Could you check a few things on this model? Use its own coordinates, in mm. Face numbers are marked on the shaded views. A direction names the side the tool comes from. Round coordinates to 2 decimals unless told otherwise and drop trailing zeros. Loops run counter-clockwise (first coordinate to the right, second up) from the corner with the lowest first, then second, coordinate; pieces in that order, holes last.
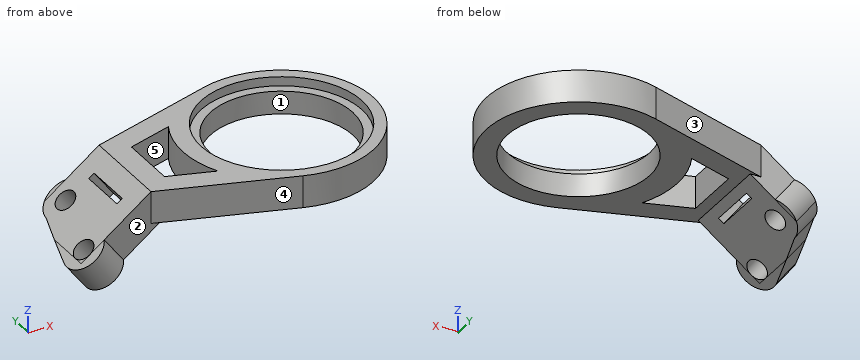
from build123d import *

# Parameters (mm, degrees)
SKETCH_1_R           = 7.75
EXTRUDE_1_DEPTH      = 3.5
SKETCH_2_R           = 8.75
CUT_EXTRUDE_1_DEPTH  = 1
EXTRUDE_2_DEPTH      = 5
SKETCH_8_W           = 0.720416832
SKETCH_8_H           = 5.4
CUT_EXTRUDE_6_DEPTH  = 26.612556655
EXTRUDE_6_DEPTH      = 3.5
SKETCH_4_9_R         = 1.15
CUT_EXTRUDE_9_DEPTH  = 27.034467236
CUT_EXTRUDE_10_DEPTH = 3.5


with BuildPart() as part:
    # 草图1 → 凸台-拉伸1 (new body)
    with BuildSketch(Plane.XY):
        with BuildLine():
            Line((-3.074847287, 9.515530157), (-17.048765133, 5))
            Line((-17.048765133, 5), (-17.048765133, -5))
            Line((-17.048765133, -5), (-3.074847287, -9.515530157))
            ThreePointArc((-3.074847287, -9.515530157), (10, 0), (-3.074847287, 9.515530157))
        make_face()
        Circle(SKETCH_1_R, mode=Mode.SUBTRACT)
        with BuildLine():
            Line((-14.548765133, 3.180565718), (-14.548765133, -3.180565718))
            Line((-14.548765133, -3.180565718), (-9.63448381, -4.768566002))
            ThreePointArc((-9.63448381, -4.768566002), (-10.75, 0), (-9.63448381, 4.768566002))
            Line((-9.63448381, 4.768566002), (-14.548765133, 3.180565718))
        make_face(mode=Mode.SUBTRACT)
    extrude(amount=EXTRUDE_1_DEPTH)

    # 草图2 → 切除-拉伸1 (cut)
    with BuildSketch(Plane.XY.offset(3.5)):
        Circle(SKETCH_2_R)
    extrude(amount=-CUT_EXTRUDE_1_DEPTH, mode=Mode.SUBTRACT)

    # 草图3 → 凸台-拉伸2 (add, symmetric)
    with BuildSketch(Plane(origin=(0, 0, 0), x_dir=(1, 0, 0), z_dir=(0, 1, 0))):
        Polygon((-17.048765133, -3.5), (-24.66318775, 2.214797011), (-22.562251427, 5.014094523), (-15.881448124, 0), align=None)
    extrude(amount=EXTRUDE_2_DEPTH, both=True)

    # 草图8 → 切除-拉伸6 (cut, through all)
    with BuildSketch(Plane(origin=(-7.82335713, 0, 10.423878111), x_dir=(0.7997992893547787, 0, 0.6002675209834286), z_dir=(-0.6002675209834286, 0, 0.7997992893547787))):
        with Locations((-14.194862331, 0)):
            Rectangle(SKETCH_8_W, SKETCH_8_H)
    extrude(amount=-CUT_EXTRUDE_6_DEPTH, mode=Mode.SUBTRACT)

    # 草图4 → 凸台-拉伸6 (add)
    with BuildSketch(Plane(origin=(-7.82335713, 0, 10.423878111), x_dir=(0.7997992893547787, 0, 0.6002675209834286), z_dir=(-0.6002675209834286, 0, 0.7997992893547787))):
        with BuildLine():
            Line((-19.939913719, 3.705712142), (-22.099126281, -3.159985282))
            ThreePointArc((-22.099126281, -3.159985282), (-20.830616239, -5.955555875), (-17.913212318, -5))
            Line((-17.913212318, -5), (-17.348837919, 1.241173708))
            Line((-17.348837919, 1.241173708), (-16.116035743, 2.269506831))
            Line((-16.116035743, 2.269506831), (-16.116035743, 5))
            ThreePointArc((-16.116035743, 5), (-18.356590206, 5.323726244), (-19.939913719, 3.705712142))
        make_face()
    extrude(amount=-EXTRUDE_6_DEPTH)

    # 草图4<9> → 切除-拉伸9 (cut, through all)
    with BuildSketch(Plane(origin=(-7.82335713, 0, 10.423878111), x_dir=(0.7997992893547787, 0, 0.6002675209834286), z_dir=(-0.6002675209834286, 0, 0.7997992893547787))):
        with Locations((-17.555070747, 2.955696144)):
            Circle(SKETCH_4_9_R)
        with Locations((-19.905070747, -3.85)):
            Circle(SKETCH_4_9_R)
    extrude(amount=-CUT_EXTRUDE_9_DEPTH, mode=Mode.SUBTRACT)

    # 草图9 → 切除-拉伸10 (cut)
    with BuildSketch(Plane(origin=(-7.82335713, 0, 10.423878111), x_dir=(0.7997992893547787, 0, 0.6002675209834286), z_dir=(-0.6002675209834286, 0, 0.7997992893547787))):
        with BuildLine():
            Line((-21.055070747, 0.15982191), (-20.046766168, 3.15929852))
            ThreePointArc((-20.046766168, 3.15929852), (-19.725256431, 4.196781997), (-18.994105751, 5))
            Line((-18.994105751, 5), (-18.994105751, 5.471830363))
            Line((-18.994105751, 5.471830363), (-21.906262893, 5.471830363))
            Line((-21.906262893, 5.471830363), (-21.906262893, 0.15982191))
            Line((-21.906262893, 0.15982191), (-21.055070747, 0.15982191))
        make_face()
    extrude(amount=-CUT_EXTRUDE_10_DEPTH, mode=Mode.SUBTRACT)


solid = part.part
Item 1: If I drill on line 1 along X through (y, z) = (0, 2.05); line 2 along Y through (x, z) = (0, 1); line 3 along X through (y, z) = (0.75, 1.5), over which ranges is the centre line in solid material (lowest first)?
Results list:
line 1: x = -18.84 to -14.55, -10.75 to -7.75, 7.75 to 10
line 2: y = -10 to -7.75, 7.75 to 10
line 3: x = -19.71 to -19.32, -18.42 to -14.55, -10.72 to -7.71, 7.71 to 9.97
Item 2: Will these pins go through, and if not, where does the flat tip stop? pin 1 (6 mm diameter, centred on x = -8.5, y = 3.5, fed in from -Z); pin 2 (3 mm diameter, centred on x = -18, z = 0, fed in from -Y); pin 3 (10 mm diameter, centred on x = -12.5, y = 0.5, fed in from +Z); pin 4 (1.5 mm diameter, centred on x = -18, z = -4, fed in from +Y).
Results list:
pin 1: stops at z = 0
pin 2: stops at y = -5.18
pin 3: stops at z = 3.5
pin 4: passes through
Item 3: If we section it at A-A, the plane x = 0: Please give me the cut outline in (y, z), then the cut area to 4 significant figures.
Results list:
outline: (-10, 0) - (-7.75, 0) - (-7.75, 2.5) - (-8.75, 2.5) - (-8.75, 3.5) - (-10, 3.5) - close; (7.75, 0) - (10, 0) - (10, 3.5) - (8.75, 3.5) - (8.75, 2.5) - (7.75, 2.5) - close
area: 13.75 mm2
Item 4: If we section it at C-C, the plane x = -13: Please give me the cut outline in (y, z).
Results list:
outline: (-6.31, 0) - (-3.68, 0) - (-3.68, 3.5) - (-6.31, 3.5) - close; (3.68, 0) - (6.31, 0) - (6.31, 3.5) - (3.68, 3.5) - close
Item 5: For the marked faces 4 and 5, which set-ups out of +Z, -Z, +X, -X, +Y, -Y let a thin tool reach every point of the face, with its end or its side?
Results list:
face 4: +Z, -Z, -X, -Y
face 5: +Z, -Z
Item 6: We'd pull the mould along Y, two halves only. Please class the marked faces 1, 2 and 3: released by +Y, released by -Y, zero draft, split by the parting line, or undercut.
Results list:
face 1: undercut
face 2: released by -Y
face 3: released by +Y
Item 7: If we section it at B-B, the plane y = -4.25: Please give me the cut outline in (x, z), then the cut area to 3 significant figures.
Results list:
outline: (-25.55, -2.88) - (-23.45, -5.68) - (-22.5, -4.97) - (-24.61, -2.17) - close; (-22.88, -0.88) - (-20.78, -3.68) - (-15.88, 0) - (-11.24, 0) - (-11.24, 3.5) - (-17.05, 3.5) - close; (-9.87, 0) - (-6.48, 0) - (-6.48, 2.5) - (-7.65, 2.5) - (-7.65, 3.5) - (-9.87, 3.5) - close; (6.48, 0) - (9.05, 0) - (9.05, 3.5) - (7.65, 3.5) - (7.65, 2.5) - (6.48, 2.5) - close
area: 64.5 mm2
